Autodesk Inventor part; units mm, degrees
ref_plane "YZ Plane" through (0, 0, 0) normal (1, 0, 0) x (0, 1, 0)
ref_plane "XZ Plane" through (0, 0, 0) normal (0, 1, 0) x (-1, 0, 0)
ref_plane "XY Plane" through (0, 0, 0) normal (0, 0, 1) x (1, 0, 0)
sketch "Sketch1" plane through (0, 0, 0) normal (1, 0, 0) x (0, 1, 0)
  line L0 (4.7625, 5.5372) -> (4.7625, -5.5372)
  line L1 (4.7625, 5.5372) -> (12.7, 5.5372)
  line L2 (12.7, 5.5372) -> (15.367, 2.8702)
  line L3 (15.367, -2.8702) -> (12.7, -5.5372)
  line L4 (12.7, -5.5372) -> (4.7625, -5.5372)
  line L5 (4.7625, 0) -> (0, 0) construction
  line L6 (4.7625, 0) -> (12.3952, 0) construction
  line L7 (15.367, 2.8702) -> (13.0048, 0.508)
  line L8 (13.0048, -0.508) -> (15.367, -2.8702)
  line L9 (13.0048, 0.508) -> (12.3952, 0.508)
  line L10 (12.3952, 0.508) -> (12.3952, -0.508)
  line L11 (12.3952, -0.508) -> (13.0048, -0.508)
  line L12 (0, -5.4393) -> (0, 5.4393) construction
  line L13 (12.7, 5.5372) -> (12.7, 0.508) construction
  dimension "d0" = 4.7625
  dimension "d1" = 12.7
  dimension "d3" = 1.016
  dimension "d4" = 11.0744
  dimension "d6" = 15.367
  dimension "d7" = 5.7404
revolve "Revolution1" add sketch "Sketch1" angle 360 about axis through (0, 0, -5.4393) along (0, 0, 1)
properties part number "roller" material "Steel, Alloy"
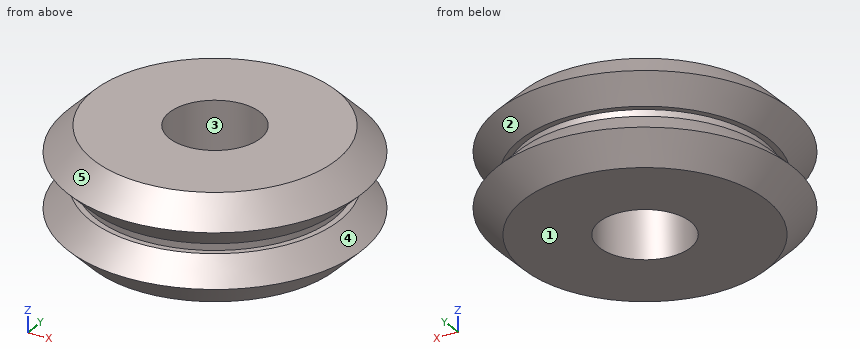
Check sheet for the modelled part. Datum: model origin and axes. Units: mm. Face numbers are marked on the shaded views. A direction names the side the tool comes from. Round coordinates to 2 decimals unless told otherwise and drop trailing zeros. Write each loop counter-clockwise with the first axis right and the second up, starting at its lowest first coordinate (ties: lowest second). Pieces come first, ordered by that corner, then holes. Notation, with made-up numbers: (27, -12.75) -> (60, -12.75) arc R16 ccw to (60, 10.25) -> close; hole circle Ø9 at (-10, 51.5). An arc over 180 degrees is marked (long way). Put each result on its own line as item: value.
(1) Tool access check on the marked faces 4 and 5. Record the directions out of +Z, -Z, +X, -X, +Y, -Y that give a thin tool (end or side, any length) a straight path to the whole face; none if there is none.
Values found:
face 4: none
face 5: +Z
(2) Mould release check, pull along X, two halves, no side actions. Record for the marked faces 1, 2 and 3: released by +X, released by -X, zero draft, split by the parting line, or undercut.
Values found:
face 1: zero draft
face 2: split by the parting line
face 3: undercut
(3) Sectioned sample at C-C (z = 4.75). Enter the section's corners in (x, y) (1 decimal), plus the area to 3 significant figures.
Values found:
outline: circle Ø27 at (0, 0); hole circle Ø9.5 at (0, 0)
area: 500 mm^2
(4) Material ranges on line 1 (X direction, y = 0, z = 0); line 2 (X direction, y = -1, z = -4); line 3 (Y direction, x = 2, z = 1.5), recorded low to high.
Values found:
line 1: x = -12.4 to -4.76, 4.76 to 12.4
line 2: x = -14.2 to -4.66, 4.66 to 14.2
line 3: y = -13.85 to -4.32, 4.32 to 13.85
(5) Go/stop test with flat-tipped pins: pin 1 Ø5.5 at (x, y) = (0, 0) entering from +Z; pin 2 Ø6 at (x, z) = (-10, -3) entering from -Y; pin 3 Ø1 at (x, z) = (5, 0.5) entering from -Y; pin 4 Ø5 at (x, z) = (-11.5, -1) entering from -Y. Record where each tip stops, or that it passes through.
Values found:
pin 1: passes through
pin 2: stops at y = -13.68
pin 3: stops at y = -12.57
pin 4: stops at y = -11.8
(6) Sectioned sample at A-A (x = 0). Enter the section's corners in (y, z).
Values found:
outline: (-15.37, -2.87) -> (-12.7, -5.54) -> (-4.76, -5.54) -> (-4.76, 5.54) -> (-12.7, 5.54) -> (-15.37, 2.87) -> (-13, 0.51) -> (-12.4, 0.51) -> (-12.4, -0.51) -> (-13, -0.51) -> close; (4.76, -5.54) -> (12.7, -5.54) -> (15.37, -2.87) -> (13, -0.51) -> (12.4, -0.51) -> (12.4, 0.51) -> (13, 0.51) -> (15.37, 2.87) -> (12.7, 5.54) -> (4.76, 5.54) -> close
